Job drawing, mm, ordinate dimensions from the low corner. One solid piece. A direction names the side the tool comes from. Give positions to 0.01 mm unless a question says otherwise; leave off trailing zeros. Order: outer loops, then holes, each group sorted by start corner. A loop starts at its lowest first (then second) coordinate and runs counter-clockwise, first axis right, second up. Notation, with made-up numbers: (71.5, -4) - (115.5, -4) arc R9 ccw to (115.5, 7) - close; hole circle Ø6 at (-26.75, 30). An arc over 180 degrees is marked (long way). One line per item, written item: value.
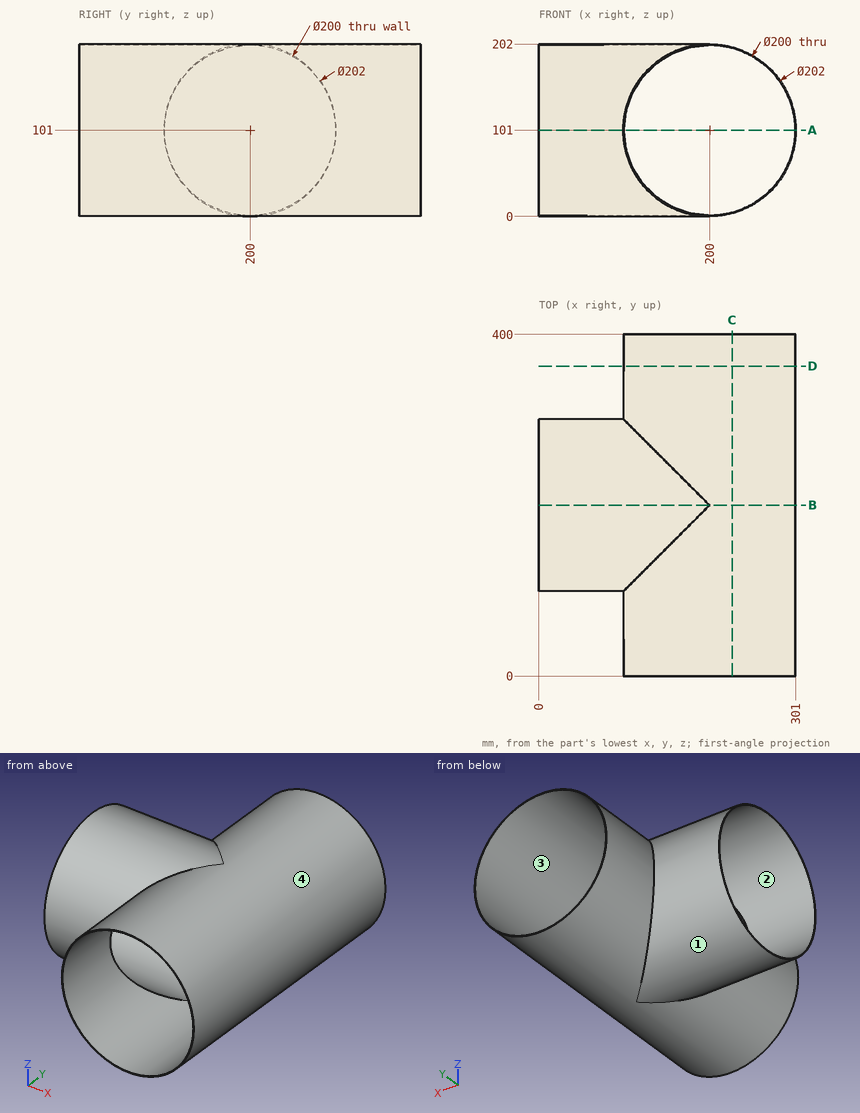
1) Slice it at A-A on z = 101. Write the cut outline in (x, y).
Answer:
outline: (0, 99) - (99, 99) - (99, 0) - (100, 0) - (100, 100) - (0, 100) - close; (0, 300) - (100, 300) - (100, 400) - (99, 400) - (99, 301) - (0, 301) - close; (300, 0) - (301, 0) - (301, 400) - (300, 400) - close
2) Which spindle directions (+Z, -Z, +X, -X, +Y, -Y) get a long thin tool onto all of the face, cutting with end or side? Do the marked faces 3 and 4. Say none if no direction does.
Answer:
face 3: +Y, -Y
face 4: none
3) Slice it at D-D on y = 363. Write the cut outline in (x, z).
Answer:
outline: circle Ø202 at (200, 101); hole circle Ø200 at (200, 101)
4) Two-plate mould, pull along Y, no slides. Class the marked faces 1 and 2: pulls with the +Y half, pulls with the -Y half, needs draft (parallel to the pull), parting line crosses it, or undercut.
Answer:
face 1: parting line crosses it
face 2: undercut
5) Slice it at B-B on y = 200. Write the cut outline in (x, z).
Answer:
outline: (0, 0) - (200, 0) arc R101 ccw to (200, 202) - (0, 202) - (0, 201) - (200, 201) arc R100 cw to (200, 1) - (0, 1) - close
6) Slice it at C-C on x = 226.5. Write the cut outline in (y, z), then the cut area to 3 significant figures.
Answer:
outline: (0, 3.54) - (400, 3.54) - (400, 4.58) - (0, 4.58) - close; (0, 197.42) - (400, 197.42) - (400, 198.46) - (0, 198.46) - close
area: 829 mm2
7) Drop flat-ended pins along their axis: P1, Ø10, axis at x = 167.5, y = 174.5, coming from the +Z side; P2, Ø5, axis at y = 261.5, z = 47.5, coming from the +X side; P3, Ø12, axis at y = 77.5, z = 100, coming from the -X side. Give the stop position or say it passes through.
Answer:
P1: stops at z = 199.9
P2: stops at x = 287.18
P3: stops at x = 99
8) Wall check: line 1 along Y through (x, z) = (94, 101); line 2 along Z through (x, y) = (138, 200); line 3 along X through (y, z) = (117.5, 104). Give the ranges that are in metal, low to high. Write a range as [from, to].
Answer:
line 1: y = [99, 100], [300, 301]
line 2: z = [0, 1], [201, 202]
line 3: x = [299.95, 300.96]
